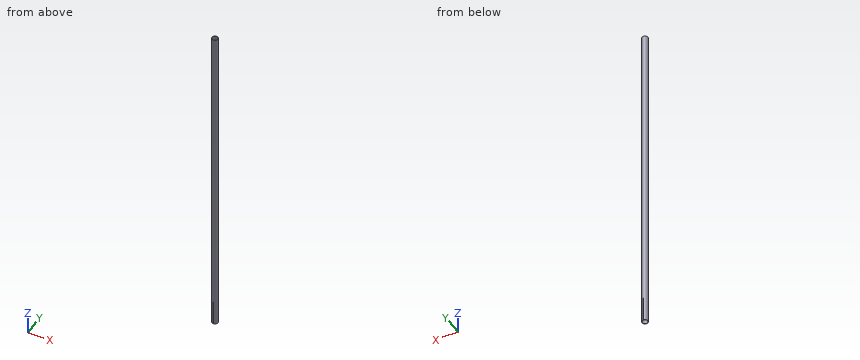
```python
from build123d import *

# Parameters (mm, degrees)
SKETCH1_R           = 17.46
SKETCH1_R_2         = 15
BOSS_EXTRUDE1_DEPTH = 1828.8
SKETCH4_W           = 2.08
SKETCH4_H           = 50
CUT_EXTRUDE2_DEPTH  = 141


with BuildPart() as part:
    # Sketch1 → Boss-Extrude1 (new body)
    with BuildSketch(Plane.XY):
        Circle(SKETCH1_R)
        Circle(SKETCH1_R_2, mode=Mode.SUBTRACT)
    extrude(amount=BOSS_EXTRUDE1_DEPTH)

    # Sketch4 → Cut-Extrude2 (cut)
    with BuildSketch(Plane.XY):
        Rectangle(SKETCH4_W, SKETCH4_H)
    extrude(amount=CUT_EXTRUDE2_DEPTH, mode=Mode.SUBTRACT)


solid = part.part
```
Model file for the job. Use its own axes, mm. Round coordinates to 2 decimals unless told otherwise and drop trailing zeros. Order: outer loops, then holes, each group sorted by start corner. A loop starts at its lowest first (then second) coordinate and runs counter-clockwise, first axis right, second up. Notation, with made-up numbers: (40.25, 10.5) -> (81.25, 10.5) arc R33 ccw to (81.25, 41.5) -> close; hole circle Ø4 at (-24.75, 68). An arc over 180 degrees is marked (long way). Use one line per item in the form item = value.
Item 1: Drill centre lines: line 1 (X direction, y = 0, z = 1454); line 2 (X direction, y = 2.5, z = 1113.5). Where is each one in solid material? Low to high.
Returned:
line_1 = -17.46 to -15, 15 to 17.46
line_2 = -17.28 to -14.79, 14.79 to 17.28
Item 2: Cut at C-C, the plane z = 834. Write the cut outline in (x, y), and give its area (3 significant figures).
Returned:
outline = circle Ø34.92 at (0, 0); hole circle Ø30 at (0, 0)
area = 251 mm^2
Item 3: Cut at B-B, the plane x = 8.5. Write the cut outline in (y, z).
Returned:
outline = (-15.25, 0) -> (-12.36, 0) -> (-12.36, 1828.8) -> (-15.25, 1828.8) -> close; (12.36, 0) -> (15.25, 0) -> (15.25, 1828.8) -> (12.36, 1828.8) -> close
Item 4: Flat gauge pins, fed straight in: pin 1 Ø0.7 at (y, z) = (-16.5, 35.5) entering from +X; pin 2 Ø3 at (x, z) = (4.5, 1201) entering from -Y; pin 3 Ø8 at (x, z) = (-6, 1254.5) entering from -Y. Where does each tip first touch, or does it go through?
Returned:
pin_1 = 6.64
pin_2 = -17.2
pin_3 = -17.35
Item 5: Cut at A-A, the plane y = 0. Write the cut outline in (x, z), and give its area (3 significant figures).
Returned:
outline = (-17.46, 0) -> (-15, 0) -> (-15, 1828.8) -> (-17.46, 1828.8) -> close; (15, 0) -> (17.46, 0) -> (17.46, 1828.8) -> (15, 1828.8) -> close
area = 9,000 mm^2
